Input: part model. Units: mm. Frame: model coordinates. Face numbers are marked on the shaded views. A direction names the side the tool comes from. Round coordinates to 2 decimals unless told otherwise and drop trailing zeros. Write each loop counter-clockwise with the first axis right and the second up, starting at its lowest first coordinate (ties: lowest second). Pieces come first, ordered by that corner, then holes. Notation, with made-up numbers: M 15.25,34 L 23.25,34 A19 cw 23.25,40 Z; hole C 70,-12 d11. An arc over 180 degrees is marked long. Answer as CSV lines item,"result". Start each with the question number.
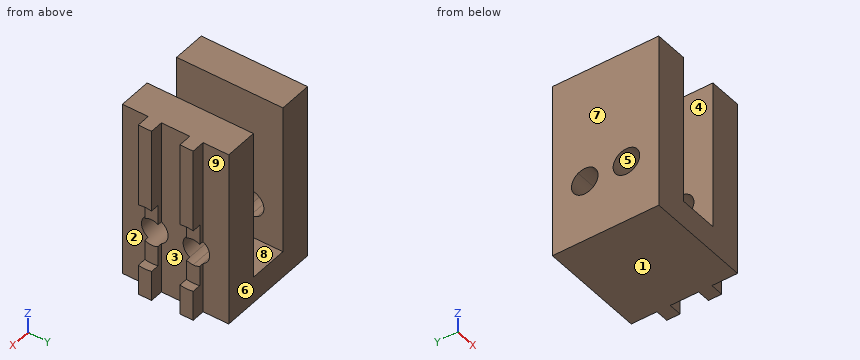
```python
from build123d import *

# Parameters (mm, degrees)
BOSS_EXTRUDE1_DEPTH = 20
SKETCH2_W           = 4.5
SKETCH2_H           = 12
CUT_EXTRUDE1_DEPTH  = 17
SKETCH3_R           = 1.5
CUT_EXTRUDE2_DEPTH  = 1
SKETCH3_3_R         = 1.5
CUT_EXTRUDE3_DEPTH  = 27.949025956


with BuildPart() as part:
    # Sketch1 → Boss-Extrude1 (new body)
    with BuildSketch(Plane.XY):
        Polygon((12, 9.1), (13.5, 9.1), (13.5, 7.6), (12, 7.6), (12, 4.4), (13.5, 4.4), (13.5, 2.9), (12, 2.9), (12, 0), (0, 0), (0, 12), (12, 12), align=None)
    extrude(amount=BOSS_EXTRUDE1_DEPTH)

    # Sketch2 → Cut-Extrude1 (cut)
    with BuildSketch(Plane.XY.offset(20)):
        with Locations((6, 6)):
            Rectangle(SKETCH2_W, SKETCH2_H)
    extrude(amount=-CUT_EXTRUDE1_DEPTH, mode=Mode.SUBTRACT)

    # Sketch3 → Cut-Extrude2 (cut)
    # profile 1 of 6: a face of its own
    with BuildSketch(Plane(origin=(13.5, 0, 0), x_dir=(0, 0, -1), z_dir=(1, 0, 0))):
        with BuildLine():
            Line((-5.700961894, 7.6), (-3.42788578, 7.6))
            ThreePointArc((-3.42788578, 7.6), (-3.35, 8.35), (-3.42788578, 9.1))
            Line((-3.42788578, 9.1), (-5.700961894, 9.1))
            ThreePointArc((-5.700961894, 9.1), (-5.551111261, 8.738228568), (-5.5, 8.35))
            ThreePointArc((-5.5, 8.35), (-5.551111261, 7.961771432), (-5.700961894, 7.6))
        make_face()
    # profile 2 of 6: a face of its own
    with BuildSketch(Plane(origin=(13.5, 0, 0), x_dir=(0, 0, -1), z_dir=(1, 0, 0))):
        with BuildLine():
            ThreePointArc((-10.57211422, 9.1), (-10.65, 8.35), (-10.57211422, 7.6))
            Line((-10.57211422, 7.6), (-8.299038106, 7.6))
            ThreePointArc((-8.299038106, 7.6), (-8.5, 8.35), (-8.299038106, 9.1))
            Line((-8.299038106, 9.1), (-10.57211422, 9.1))
        make_face()
    # profile 3 of 6: a face of its own
    with BuildSketch(Plane(origin=(13.5, 0, 0), x_dir=(0, 0, -1), z_dir=(1, 0, 0))):
        with BuildLine():
            ThreePointArc((-9.792848009, 6), (-7, 0), (-4.207151991, 6))
            ThreePointArc((-4.207151991, 6), (-3.718508564, 6.751777876), (-3.42788578, 7.6))
            Line((-3.42788578, 7.6), (-5.700961894, 7.6))
            ThreePointArc((-5.700961894, 7.6), (-7, 6.85), (-8.299038106, 7.6))
            Line((-8.299038106, 7.6), (-10.57211422, 7.6))
            ThreePointArc((-10.57211422, 7.6), (-10.281491436, 6.751777876), (-9.792848009, 6))
        make_face()
        with Locations((-7, 3.65)):
            Circle(SKETCH3_R, mode=Mode.SUBTRACT)
    # profile 4 of 6: a face of its own
    with BuildSketch(Plane(origin=(13.5, 0, 0), x_dir=(0, 0, -1), z_dir=(1, 0, 0))):
        with BuildLine():
            Line((-5.700961894, 9.1), (-3.42788578, 9.1))
            ThreePointArc((-3.42788578, 9.1), (-7, 12), (-10.57211422, 9.1))
            Line((-10.57211422, 9.1), (-8.299038106, 9.1))
            ThreePointArc((-8.299038106, 9.1), (-7, 9.85), (-5.700961894, 9.1))
        make_face()
    # profile 5 of 6: a face of its own
    with BuildSketch(Plane(origin=(13.5, 0, 0), x_dir=(0, 0, -1), z_dir=(1, 0, 0))):
        with BuildLine():
            Line((-5.700961894, 7.6), (-3.42788578, 7.6))
            ThreePointArc((-3.42788578, 7.6), (-3.35, 8.35), (-3.42788578, 9.1))
            Line((-3.42788578, 9.1), (-5.700961894, 9.1))
            ThreePointArc((-5.700961894, 9.1), (-5.551111261, 8.738228568), (-5.5, 8.35))
            ThreePointArc((-5.5, 8.35), (-5.551111261, 7.961771432), (-5.700961894, 7.6))
        make_face()
    # profile 6 of 6: a face of its own
    with BuildSketch(Plane(origin=(13.5, 0, 0), x_dir=(0, 0, -1), z_dir=(1, 0, 0))):
        with BuildLine():
            ThreePointArc((-10.57211422, 9.1), (-10.65, 8.35), (-10.57211422, 7.6))
            Line((-10.57211422, 7.6), (-8.299038106, 7.6))
            ThreePointArc((-8.299038106, 7.6), (-8.5, 8.35), (-8.299038106, 9.1))
            Line((-8.299038106, 9.1), (-10.57211422, 9.1))
        make_face()
    extrude(amount=-CUT_EXTRUDE2_DEPTH, mode=Mode.SUBTRACT)

    # Sketch3_3 → Cut-Extrude3 (cut, through all)
    with BuildSketch(Plane(origin=(13.5, 0, 0), x_dir=(0, 0, -1), z_dir=(1, 0, 0))):
        with BuildLine():
            Line((-8.299038106, 7.6), (-5.700961894, 7.6))
            ThreePointArc((-5.700961894, 7.6), (-5.551111261, 7.961771432), (-5.5, 8.35))
            ThreePointArc((-5.5, 8.35), (-5.551111261, 8.738228568), (-5.700961894, 9.1))
            Line((-5.700961894, 9.1), (-8.299038106, 9.1))
            ThreePointArc((-8.299038106, 9.1), (-8.5, 8.35), (-8.299038106, 7.6))
        make_face()
        with BuildLine():
            ThreePointArc((-8.299038106, 7.6), (-7, 6.85), (-5.700961894, 7.6))
            Line((-5.700961894, 7.6), (-8.299038106, 7.6))
        make_face()
        with BuildLine():
            Line((-8.299038106, 9.1), (-5.700961894, 9.1))
            ThreePointArc((-5.700961894, 9.1), (-7, 9.85), (-8.299038106, 9.1))
        make_face()
        with Locations(Location((-7, 3.65, 0), (0, 0, 30))):
            Circle(SKETCH3_3_R)
    extrude(amount=-CUT_EXTRUDE3_DEPTH, mode=Mode.SUBTRACT)


solid = part.part
```
Item 1: Draft query along X for the marked faces 6, 7, 8 and 9. Return one class per face: +X half, -X half, draft (parallel to the pull), parting line (faces both ways), or undercut.
Item 2: Pin query (flat end, axial travel): pin 1 Ø0.8 at (x, z) = (13, 13) entering from +Y; pin 2 Ø1.7 at (y, z) = (3.5, 4.5) entering from +X; pin 3 Ø1.5 at (y, z) = (11, 12) entering from +X. Return the tip coordinate at first contact, or that it passes through.
Item 3: Cut plane B-B, the plane y = 3.65. Return loops of the section in (x, z).
Item 4: Access query for the marked faces 1, 2, 3, 4 and 5. Directions: +Z, -Z, +X, -X, +Y, -Y. A direction counts if a zero-diameter tool reaches every point of the face in a straight line with its end or side. Return the directions, or none.
Item 5: Cut plane C-C, the plane z = 7. Return loops of the section in (x, y).
Item 6: Cut plane A-A, the plane z = 11. Return loops of the section in (x, y), plus the area to 3 significant figures.
Item 7: Cut plane D-D, the plane x = 3. Return loops of the section in (y, z), plus the area to 3 significant figures.
Item 8: Line query: line 1 (X direction, y = 5.25, z = 6.5); line 2 (Z direction, x = 11.35, y = 3.65); line 3 (Z direction, x = 6.25, y = 5). Output: solid intervals per line, ascending. Write a range as [from, to].
Results list:
1,face 6,"draft"
1,face 7,"-X half"
1,face 8,"undercut"
1,face 9,"+X half"
2,pin 1,"y = 9.1"
2,pin 2,"x = 12.5"
2,pin 3,"x = 12"
3,outline,"M 0,0 L 13.5,0 L 13.5,3.35 L 12.5,3.35 L 12.5,5.5 L 8.25,5.5 L 8.25,3 L 3.75,3 L 3.75,5.5 L 0,5.5 Z; M 0,8.5 L 3.75,8.5 L 3.75,20 L 0,20 Z; M 8.25,8.5 L 12.5,8.5 L 12.5,10.65 L 13.5,10.65 L 13.5,20 L 8.25,20 Z"
4,face 1,"-Z, +X, -X, +Y, -Y"
4,face 2,"+Z, -Z, +X, -Y"
4,face 3,"+Z, -Z, +X"
4,face 4,"+Z, +Y, -Y"
4,face 5,"+X, -X"
5,outline,"M 0,0 L 3.75,0 L 3.75,2.15 L 0,2.15 Z; M 0,5.15 L 3.75,5.15 L 3.75,6.85 L 0,6.85 Z; M 0,9.85 L 3.75,9.85 L 3.75,12 L 0,12 Z; M 8.25,0 L 12,0 L 12,2.15 L 8.25,2.15 Z; M 8.25,5.15 L 12,5.15 L 12,6.85 L 8.25,6.85 Z; M 8.25,9.85 L 12,9.85 L 12,12 L 8.25,12 Z"
6,outline,"M 0,0 L 3.75,0 L 3.75,12 L 0,12 Z; M 8.25,0 L 12,0 L 12,2.9 L 13.5,2.9 L 13.5,4.4 L 12,4.4 L 12,7.6 L 13.5,7.6 L 13.5,9.1 L 12,9.1 L 12,12 L 8.25,12 Z"
6,area,"94.5 mm²"
7,outline,"M 0,0 L 12,0 L 12,20 L 0,20 Z; hole C 3.65,7 d3; hole C 8.35,7 d3"
7,area,"226 mm²"
8,line 1,"[0, 3.75], [8.25, 12]"
8,line 2,"[0, 5.5], [8.5, 20]"
8,line 3,"[0, 3]"
